from build123d import *

# Parameters (mm, degrees)
SKETCH_1_R               = 35
SKETCH_1_R_2             = 25
EXTRUDE_1_DEPTH          = 10
SKETCH_2_R               = 12.5
EXTRUDE_2_DEPTH          = 10
PATTERN_CIRCULAR_1_COUNT = 5
SKETCH_3_R               = 2.5
CUT_EXTRUDE_1_DEPTH      = 54.38539126
CUT_EXTRUDE_2_DEPTH      = 10


with BuildPart() as part:
    # 草图1 → 凸台-拉伸1 (new, symmetric)
    with BuildSketch(Plane.XY):
        Circle(SKETCH_1_R)
        Circle(SKETCH_1_R_2, mode=Mode.SUBTRACT)
    extrude(amount=EXTRUDE_1_DEPTH, both=True)

    # 草图2 → 凸台-拉伸2 (add, symmetric)
    with BuildSketch(Plane.XY):
        Circle(SKETCH_2_R)
        with BuildLine():
            Line((-1.438766033, 31.712801318), (-3.859353097, 11.889297443))
            ThreePointArc((-3.859353097, 11.889297443), (0.427174783, 12.492698736), (4.662473362, 11.597902489))
            Line((4.662473362, 11.597902489), (1.678560372, 31.712801318))
            Line((1.678560372, 31.712801318), (-1.438766033, 31.712801318))
        make_face()
    extrude_2 = extrude(amount=EXTRUDE_2_DEPTH, both=True)

    # 阵列(圆周)1: 凸台-拉伸2 ×5 about axis
    pattern_circular_1_axis = Axis((0, 0, 0), (0, 0, 1))
    for i in range(1, PATTERN_CIRCULAR_1_COUNT):
        add(extrude_2.rotate(pattern_circular_1_axis, i * 360 / PATTERN_CIRCULAR_1_COUNT))

    # 草图3 → 切除-拉伸1 (cut, through all)
    with BuildSketch(Plane.XY.offset(10)):
        Circle(SKETCH_3_R)
    extrude(amount=-CUT_EXTRUDE_1_DEPTH, mode=Mode.SUBTRACT)

    # 草图4 → 切除-拉伸2 (cut)
    with BuildSketch(Plane(origin=(0, 0, -10), x_dir=(-1, 0, 0), z_dir=(0, 0, -1))):
        Polygon((0, 8), (-6.92820323, 4), (-6.92820323, -4), (0, -8), (6.92820323, -4), (6.92820323, 4), align=None)
    extrude(amount=-CUT_EXTRUDE_2_DEPTH, mode=Mode.SUBTRACT)


solid = part.part
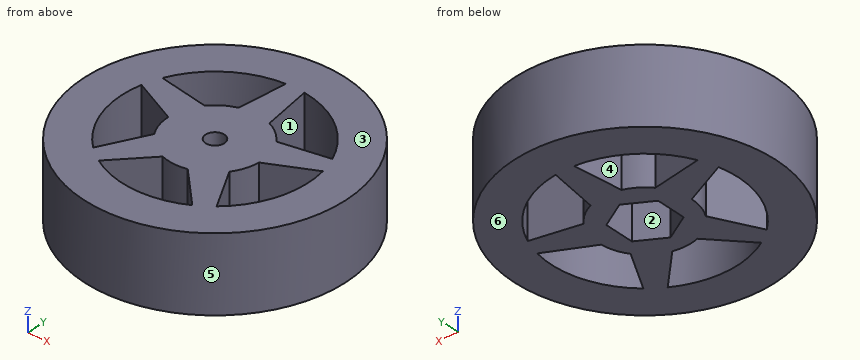
Read the model definition and answer for the solid it produces. Units are mm, in the model's axes. Face numbers are marked on the shaded views. A direction names the side the tool comes from. Round coordinates to 2 decimals unless told otherwise and drop trailing zeros. Write each loop counter-clockwise with the first axis right and the second up, starting at its lowest first coordinate (ties: lowest second). Pieces come first, ordered by that corner, then holes. Notation, with made-up numbers: (-39, -16.75) - (-13, -16.75) arc R30 ccw to (-13, 13.25) - close; hole circle Ø1 at (55, 23.25). An arc over 180 degrees is marked (long way). Use a Markdown table: item, result.
(1) Each of these flat-tipped pins is pushed along its axis until it touches: pin 1 Ø8 at (x, z) = (12, 7) entering from -Y; pin 2 Ø2 at (x, z) = (-11.5, 0.5) entering from -Y; pin 3 Ø12 at (x, z) = (-18.5, -4.5) entering from -Y; pin 4 Ø6 at (x, y) = (-20.5, -3.5) entering from +Z. Where does it stop, or does it pass through?
Reported:
| item | result |
|---|---|
| pin 1 | y = -34.07 |
| pin 2 | y = -33.39 |
| pin 3 | y = -32.69 |
| pin 4 | through |
(2) Which of the six approach directions +Z, -Z, +X, -X, +Y, -Y give full straight-line access (tool end or side, diameter ignored) to the marked faces 1, 2 and 3?
Reported:
| item | result |
|---|---|
| face 1 | +Z, -Z |
| face 2 | -Z |
| face 3 | +Z, +X, -X, +Y, -Y |
(3) The part is cut by section D-D (z = -4.75). Write down the section's boundary in (x, y), then the cut area to 3 significant figures.
Reported:
| item | result |
|---|---|
| outline | circle Ø70 at (0, 0); hole (-24.38, 5.53) arc R25 ccw to (-16.79, -18.52) - (-10.59, -6.64) arc R12.5 cw to (-12.5, 0) - close; hole (-22.8, 10.24) - (-9.59, 8.02) arc R12.5 cw to (-3.86, 11.89) - (-2.27, 24.9) arc R25 ccw to start; hole (-12.8, -21.48) arc R25 ccw to (12.43, -21.69) - (3.05, -12.12) arc R12.5 cw to (-3.87, -11.89) - close; hole (-6.93, -4) - (0, -8) - (6.93, -4) - (6.93, 4) - (0, 8) - (-6.93, 4) - close; hole (2.7, 24.85) - (4.66, 11.6) arc R12.5 cw to (10.11, 7.34) - (22.98, 9.85) arc R25 ccw to start; hole (10.11, -7.35) - (16.47, -18.81) arc R25 ccw to (24.47, 5.12) - (12.47, -0.85) arc R12.5 cw to start |
| area | 2,630 mm2 |
(4) Straight lines are drawn through the part: line 1 along Y through (x, z) = (0, 3.5); line 2 along Y through (x, z) = (5.5, 9); line 3 along X through (y, z) = (21.5, 0.75). For each, find the intervals that lie inside material, in ascending order. Write a range as [from, to].
Reported:
| item | result |
|---|---|
| line 1 | [-35, -25], [-12.5, -2.5], [2.5, 35] |
| line 2 | [-34.57, -24.39], [-14.63, 11.22], [24.39, 34.57] |
| line 3 | [-27.62, -12.76], [-2.69, 3.19], [12.76, 27.62] |
(5) The part is cut by section B-B (y = 23.5). Write down the section's boundary in (x, z), then the cut area to 3 significant figures.
Reported:
| item | result |
|---|---|
| outline | (-25.94, -10) - (-8.53, -10) - (-8.53, 10) - (-25.94, 10) - close; (-2.44, -10) - (2.9, -10) - (2.9, 10) - (-2.44, 10) - close; (8.53, -10) - (25.94, -10) - (25.94, 10) - (8.53, 10) - close |
| area | 803 mm2 |
(6) The part is cut by section A-A (z = 4.5). Write down the section's boundary in (x, y).
Reported:
| item | result |
|---|---|
| outline | circle Ø70 at (0, 0); hole (-24.38, 5.53) arc R25 ccw to (-16.79, -18.52) - (-10.59, -6.64) arc R12.5 cw to (-12.5, 0) - close; hole (-22.8, 10.24) - (-9.59, 8.02) arc R12.5 cw to (-3.86, 11.89) - (-2.27, 24.9) arc R25 ccw to start; hole (-12.8, -21.48) arc R25 ccw to (12.43, -21.69) - (3.05, -12.12) arc R12.5 cw to (-3.87, -11.89) - close; hole circle Ø5 at (0, 0); hole (2.7, 24.85) - (4.66, 11.6) arc R12.5 cw to (10.11, 7.34) - (22.98, 9.85) arc R25 ccw to start; hole (10.11, -7.35) - (16.47, -18.81) arc R25 ccw to (24.47, 5.12) - (12.47, -0.85) arc R12.5 cw to start |
(7) The mould has two halves that part along X. Classify the marked faces 4, 5 and 6: released by +X, released by -X, zero draft, split by the parting line, or undercut.
Reported:
| item | result |
|---|---|
| face 4 | undercut |
| face 5 | split by the parting line |
| face 6 | zero draft |
(8) The part is cut by section C-C (x = 17.5). Write down the section's boundary in (y, z), then the cut area to 3 significant figures.
Reported:
| item | result |
|---|---|
| outline | (-30.31, -10) - (-17.85, -10) - (-17.85, 10) - (-30.31, 10) - close; (1.65, -10) - (8.79, -10) - (8.79, 10) - (1.65, 10) - close; (17.85, -10) - (30.31, -10) - (30.31, 10) - (17.85, 10) - close |
| area | 641 mm2 |
